For this review, take the finished solid that the model builds, in its own axes (mm). Face numbers are marked on the shaded views. A direction names the side the tool comes from. Round coordinates to 2 decimals unless told otherwise and drop trailing zeros. Write each loop counter-clockwise with the first axis right and the second up, starting at its lowest first coordinate (ties: lowest second). Pieces come first, ordered by that corner, then holes. Notation, with made-up numbers: M 14,51 L 65,51 A20 ccw 65,82 Z; hole C 88.5,45 d9. An arc over 180 degrees is marked long. One line per question, with ' | ' between items.
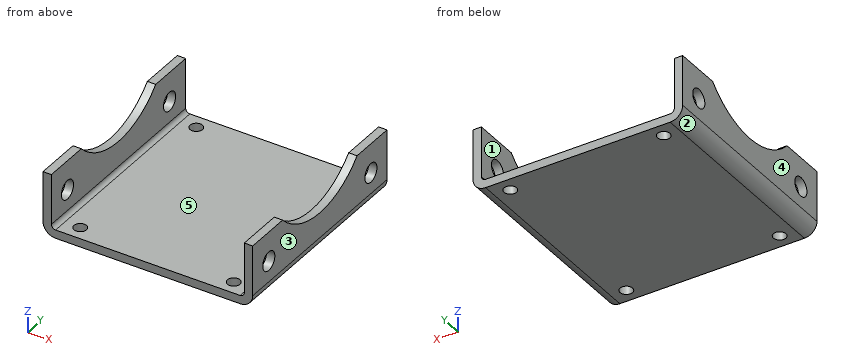
```python
from build123d import *

# Parameters (mm, degrees)
BOSS_EXTRUDE1_DEPTH = 50
SKETCH2_R           = 19
SKETCH2_R_2         = 2.25
CUT_EXTRUDE1_DEPTH  = 73.284161474
SKETCH3_R           = 1.5
CUT_EXTRUDE2_DEPTH  = 10


with BuildPart() as part:
    # Sketch1 → Boss-Extrude1 (new body)
    with BuildSketch(Plane(origin=(0, 0, 0), x_dir=(1, 0, 0), z_dir=(0, 1, 0))):
        with BuildLine():
            Line((-2, 0), (-2, 12))
            ThreePointArc((-2, 12), (-1.121320344, 14.121320344), (1, 15))
            Line((1, 15), (45, 15))
            ThreePointArc((45, 15), (47.121320344, 14.121320344), (48, 12))
            Line((48, 12), (48, 0))
            Line((48, 0), (46, 0))
            Line((46, 0), (46, 12))
            ThreePointArc((46, 12), (45.707106781, 12.707106781), (45, 13))
            Line((45, 13), (1, 13))
            ThreePointArc((1, 13), (0.292893219, 12.707106781), (0, 12))
            Line((0, 12), (0, 0))
            Line((0, 0), (-2, 0))
        make_face()
    extrude(amount=BOSS_EXTRUDE1_DEPTH)

    # Sketch2 → Cut-Extrude1 (cut, through all)
    with BuildSketch(Plane(origin=(48, 0, 0), x_dir=(0, 0, -1), z_dir=(1, 0, 0))):
        with Locations((-13, 25)):
            Circle(SKETCH2_R)
        with Locations((7, 44)):
            Circle(SKETCH2_R_2)
        with Locations((7, 6)):
            Circle(SKETCH2_R_2)
    extrude(amount=-CUT_EXTRUDE1_DEPTH, mode=Mode.SUBTRACT)

    # Sketch3 → Cut-Extrude2 (cut)
    with BuildSketch(Plane(origin=(0, 0, -15), x_dir=(-1, 0, 0), z_dir=(0, 0, -1))):
        with Locations((-41.29, 46.59)):
            Circle(SKETCH3_R)
        with Locations((-4.71, 46.59)):
            Circle(SKETCH3_R)
        with Locations((-4.71, 3.41)):
            Circle(SKETCH3_R)
        with Locations((-41.29, 3.41)):
            Circle(SKETCH3_R)
    extrude(amount=-CUT_EXTRUDE2_DEPTH, mode=Mode.SUBTRACT)


solid = part.part
```
Item 1: To check wall thickness, follow line 1 along Y through (x, z) = (41.29, -14.3); line 2 along Y through (x, z) = (-1.5, -7); line 3 along X through (y, z) = (19, -6.75). State the ranges of each line that lie inside material, in increasing order. Write a range as from..to.
Results:
line 1: 0..1.91, 4.91..45.09, 48.09..50 | line 2: 0..3.75, 8.25..41.75, 46.25..50 | line 3: -2..0, 46..48
Item 2: Take a section at D-D (y = 37). Write out the cut boundary in (x, z), then the cut area to 3 significant figures.
Results:
outline: M -2,-12 A3 ccw 1,-15 L 45,-15 A3 ccw 48,-12 L 48,-1.73 L 46,-1.73 L 46,-12 A1 cw 45,-13 L 1,-13 A1 cw 0,-12 L 0,-1.73 L -2,-1.73 Z | area: 142 mm2
Item 3: Take a section at C-C (x = 41.29). Write out the cut boundary in (y, z).
Results:
outline: M 0,-15 L 1.91,-15 L 1.91,-13 L 0,-13 Z; M 4.91,-15 L 45.09,-15 L 45.09,-13 L 4.91,-13 Z; M 48.09,-15 L 50,-15 L 50,-13 L 48.09,-13 Z
Item 4: Mouldability with a two-part tool opening along X and no side actions: class the marked faces 3, 4 and 5 as +X half, -X half, draft (parallel to the pull), parting line (faces both ways), or undercut.
Results:
face 3: +X half | face 4: -X half | face 5: undercut
Item 5: Take a section at A-A (z = -7). Write out the cut boundary in (x, y).
Results:
outline: M -2,0 L 0,0 L 0,3.75 L -2,3.75 Z; M -2,8.25 L 0,8.25 L 0,41.75 L -2,41.75 Z; M -2,46.25 L 0,46.25 L 0,50 L -2,50 Z; M 46,0 L 48,0 L 48,3.75 L 46,3.75 Z; M 46,8.25 L 48,8.25 L 48,41.75 L 46,41.75 Z; M 46,46.25 L 48,46.25 L 48,50 L 46,50 Z
Item 6: Take a section at B-B (y = 44). Write out the cut boundary in (x, z), then the cut area to 3 significant figures.
Results:
outline: M -2,-12 A3 ccw 1,-15 L 45,-15 A3 ccw 48,-12 L 48,-9.25 L 46,-9.25 L 46,-12 A1 cw 45,-13 L 1,-13 A1 cw 0,-12 L 0,-9.25 L -2,-9.25 Z; M -2,-4.75 L 0,-4.75 L 0,0 L -2,0 Z; M 46,-4.75 L 48,-4.75 L 48,0 L 46,0 Z | area: 131 mm2
Item 7: Machinability: for the marked faces 1 and 2, which of the approach directions +Z, -Z, +X, -X, +Y, -Y give a long, thin tool a straight path to every point of the face, cutting with its end or side? Answer none if there is none.
Results:
face 1: +Z, +Y, -Y | face 2: -Z, -X, +Y, -Y
Item 8: Insertion check: pin 1 Ø2.5 at (x, y) = (41.29, 46.59) entering from +Z; pin 2 Ø8 at (y, z) = (28.5, -13) entering from +X; pin 3 Ø3.5 at (x, y) = (41.29, 3.41) entering from +Z. Each pin has a flat end and moves straight along its axis. Give the tip position at first contact, or say it passes through.
Results:
pin 1: through | pin 2: x = 48 | pin 3: z = -13
